Input: part model. Units: mm. Frame: model coordinates. Face numbers are marked on the shaded views. A direction names the side the tool comes from. Give positions to 0.01 mm unless a question says otherwise; leave off trailing zeros. Loops run counter-clockwise (first coordinate to the right, second up) from the corner with the lowest first, then second, coordinate; pieces in that order, holes last. Notation, with made-up numbers: (50, 28.5) -> (69, 28.5) arc R18 ccw to (69, 45.5) -> close; hole circle Ø6 at (18, 72). An arc over 180 degrees is marked (long way). Answer as a JSON object with one key per item and string values.
```python
from build123d import *

# Parameters (mm, degrees)
PAD_DEPTH       = 40
SKETCH001_R     = 4
POCKET_DEPTH    = 2.501
SKETCH002_R     = 4
POCKET001_DEPTH = 2.501


with BuildPart() as part:
    # Sketch → Pad (new body)
    with BuildSketch(Plane.XZ):
        Polygon((0, 0), (0, 40), (2.5, 40), (2.5, 2.5), (40, 2.5), (40, 0), align=None)
    extrude(amount=PAD_DEPTH)

    # Sketch001 (on Face3 of Pad) → Pocket (cut, through all)
    with BuildSketch(Plane(origin=(2.5, 0, 0), x_dir=(0, 0, 1), z_dir=(1, 0, 0))):
        with Locations((8.5, 34)):
            Circle(SKETCH001_R)
        with Locations((34, 34)):
            Circle(SKETCH001_R)
        with Locations((8.5, 6)):
            Circle(SKETCH001_R)
        with Locations((34, 6)):
            Circle(SKETCH001_R)
        with Locations((20, 20)):
            Circle(SKETCH001_R)
    extrude(amount=-POCKET_DEPTH, mode=Mode.SUBTRACT)

    # Sketch002 (on Face13 of Pocket) → Pocket001 (cut, through all)
    with BuildSketch(Plane(origin=(0, 0, 2.5), x_dir=(-1, 0, 0), z_dir=(0, 0, 1))):
        with Locations((-8.5, 6)):
            Circle(SKETCH002_R)
        with Locations((-34, 6)):
            Circle(SKETCH002_R)
        with Locations((-8.5, 34)):
            Circle(SKETCH002_R)
        with Locations((-34, 34)):
            Circle(SKETCH002_R)
        with Locations((-20, 20)):
            Circle(SKETCH002_R)
    extrude(amount=-POCKET001_DEPTH, mode=Mode.SUBTRACT)


solid = part.part
```
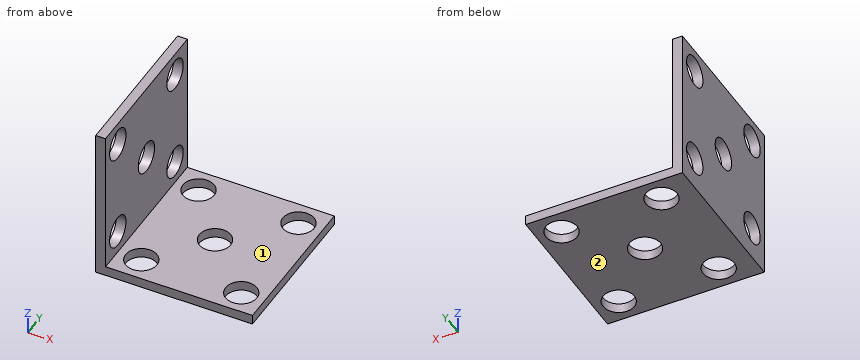
Q1. Section A-A, the plane y = -6. Return the cut outline in (x, z).
Evaluation:
{"outline": "(0, 0) -> (4.5, 0) -> (4.5, 2.5) -> (2.5, 2.5) -> (2.5, 4.5) -> (0, 4.5) -> close; (0, 12.5) -> (2.5, 12.5) -> (2.5, 30) -> (0, 30) -> close; (0, 38) -> (2.5, 38) -> (2.5, 40) -> (0, 40) -> close; (12.5, 0) -> (30, 0) -> (30, 2.5) -> (12.5, 2.5) -> close; (38, 0) -> (40, 0) -> (40, 2.5) -> (38, 2.5) -> close"}
Q2. Section B-B, the plane x = 20. Return the cut outline in (y, z), then the cut area to 3 significant figures.
Evaluation:
{"outline": "(-40, 0) -> (-24, 0) -> (-24, 2.5) -> (-40, 2.5) -> close; (-16, 0) -> (0, 0) -> (0, 2.5) -> (-16, 2.5) -> close", "area": "80.0 mm2"}
Q3. Pin query (flat end, axial travel): pin 1 (8 mm diameter, centred on y = -23.5, z = 22, fed in from +X); pin 2 (19 mm diameter, centred on x = 24.5, y = -11, fed in from +Z); pin 3 (10 mm diameter, centred on x = 16, y = -17, fed in from -Z). Return the tip coordinate at first contact, or that it passes through.
Evaluation:
{"pin 1": "stops at x = 2.5", "pin 2": "stops at z = 2.5", "pin 3": "stops at z = 0"}
Q4. Access query for the marked faces 1 and 2. Directions: +Z, -Z, +X, -X, +Y, -Y. A direction counts if a zero-diameter tool reaches every point of the face in a straight line with its end or side. Return the directions, or none.
Evaluation:
{"face 1": "+Z, +X, +Y, -Y", "face 2": "-Z, +X, -X, +Y, -Y"}
Q5. Section D-D, the plane x = 34. Return the cut outline in (y, z).
Evaluation:
{"outline": "(-40, 0) -> (-38, 0) -> (-38, 2.5) -> (-40, 2.5) -> close; (-30, 0) -> (-10, 0) -> (-10, 2.5) -> (-30, 2.5) -> close; (-2, 0) -> (0, 0) -> (0, 2.5) -> (-2, 2.5) -> close"}
Q6. Ray query, line 1 along Z through (x, y) = (1.85, -34); line 2 along Y through (x, z) = (1.95, 34). Return the intervals inside material, ascending.
Evaluation:
{"line 1": "z = 0 to 4.5, 12.5 to 30, 38 to 40", "line 2": "y = -40 to -38, -30 to -10, -2 to 0"}
Q7. Section C-C, the plane z = 34. Return the cut outline in (x, y), then the cut area to 3 significant figures.
Evaluation:
{"outline": "(0, -40) -> (2.5, -40) -> (2.5, -38) -> (0, -38) -> close; (0, -30) -> (2.5, -30) -> (2.5, -10) -> (0, -10) -> close; (0, -2) -> (2.5, -2) -> (2.5, 0) -> (0, 0) -> close", "area": "60.0 mm2"}
